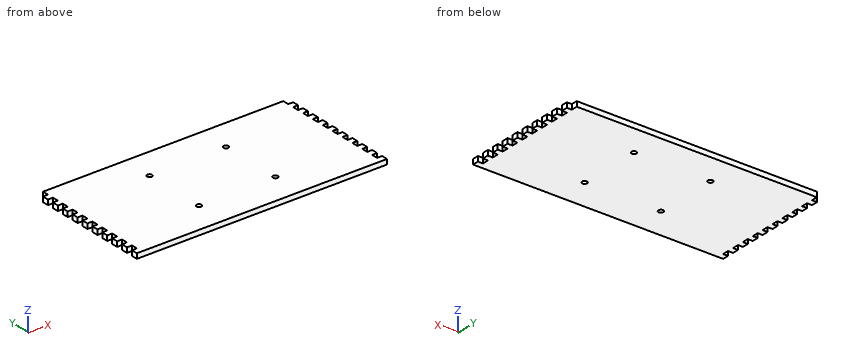
Solid Edge part; units mm, degrees
sketch "Sketch1" plane through (0, 0, 0) normal (0, 0, 1) x (1, 0, 0)
  line L0 (-100, -50) -> (100, -50)
  line L1 (100, -50) -> (100, 50)
  line L2 (100, 50) -> (-100, 50)
  line L3 (-100, 50) -> (-100, -50)
  dimension "D1" = 100
  dimension "D2" = 100
extrude "Protrusion1" add sketch "Sketch1" along normal blind 4
sketch "Sketch2" plane through (14.6999, -33.2226, 4) normal (0, 0, 1) x (1, 0, 0)
  line L0 (-114.6999, 68.2226) -> (-110.6999, 68.2226)
  line L1 (-110.6999, 68.2226) -> (-110.6999, 73.2226)
  line L2 (-110.6999, 73.2226) -> (-114.6999, 73.2226)
  line L3 (-114.6999, 73.2226) -> (-114.6999, 68.2226)
  line L4 (-114.6999, 58.2226) -> (-110.6999, 58.2226)
  line L5 (-110.6999, 58.2226) -> (-110.6999, 63.2226)
  line L6 (-110.6999, 63.2226) -> (-114.6999, 63.2226)
  line L7 (-114.6999, 63.2226) -> (-114.6999, 58.2226)
  line L8 (-114.6999, 48.2226) -> (-110.6999, 48.2226)
  line L9 (-110.6999, 48.2226) -> (-110.6999, 53.2226)
  line L10 (-110.6999, 53.2226) -> (-114.6999, 53.2226)
  line L11 (-114.6999, 53.2226) -> (-114.6999, 48.2226)
  line L12 (-114.6999, 38.2226) -> (-110.6999, 38.2226)
  line L13 (-110.6999, 38.2226) -> (-110.6999, 43.2226)
  line L14 (-110.6999, 43.2226) -> (-114.6999, 43.2226)
  line L15 (-114.6999, 43.2226) -> (-114.6999, 38.2226)
  line L16 (-114.6999, 28.2226) -> (-110.6999, 28.2226)
  line L17 (-110.6999, 28.2226) -> (-110.6999, 33.2226)
  line L18 (-110.6999, 33.2226) -> (-114.6999, 33.2226)
  line L19 (-114.6999, 33.2226) -> (-114.6999, 28.2226)
  line L20 (-114.6999, 18.2226) -> (-110.6999, 18.2226)
  line L21 (-110.6999, 18.2226) -> (-110.6999, 23.2226)
  line L22 (-110.6999, 23.2226) -> (-114.6999, 23.2226)
  line L23 (-114.6999, 23.2226) -> (-114.6999, 18.2226)
  line L24 (-114.6999, 8.2226) -> (-110.6999, 8.2226)
  line L25 (-110.6999, 8.2226) -> (-110.6999, 13.2226)
  line L26 (-110.6999, 13.2226) -> (-114.6999, 13.2226)
  line L27 (-114.6999, 13.2226) -> (-114.6999, 8.2226)
  line L28 (-114.6999, -1.7774) -> (-110.6999, -1.7774)
  line L29 (-110.6999, -1.7774) -> (-110.6999, 3.2226)
  line L30 (-110.6999, 3.2226) -> (-114.6999, 3.2226)
  line L31 (-114.6999, 3.2226) -> (-114.6999, -1.7774)
  line L32 (-114.6999, -11.7774) -> (-110.6999, -11.7774)
  line L33 (-110.6999, -11.7774) -> (-110.6999, -6.7774)
  line L34 (-110.6999, -6.7774) -> (-114.6999, -6.7774)
  line L35 (-114.6999, -6.7774) -> (-114.6999, -11.7774)
  line L36 (-114.6999, 78.2226) -> (-110.6999, 78.2226)
  line L37 (-110.6999, 78.2226) -> (-110.6999, 83.2226)
  line L38 (-110.6999, 83.2226) -> (-114.6999, 83.2226)
  line L39 (-114.6999, 83.2226) -> (-114.6999, 78.2226)
  dimension "D1" = 110.6999
  dimension "D2" = 114.6999
  dimension "D3" = 110.6999
  dimension "D4" = 110.6999
  dimension "D5" = 110.6999
  dimension "D6" = 114.6999
  dimension "D7" = 110.6999
  dimension "D8" = 110.6999
  dimension "D9" = 110.6999
  dimension "D10" = 110.6999
  dimension "D11" = 110.6999
  dimension "D12" = 110.6999
  dimension "D13" = 110.6999
  dimension "D14" = 110.6999
  dimension "D15" = 110.6999
  dimension "D16" = 110.6999
  dimension "D17" = 110.6999
  dimension "D18" = 110.6999
  dimension "D19" = 110.6999
  dimension "D20" = 114.6999
  dimension "D21" = 114.6999
  dimension "D22" = 110.6999
extrude "Cutout1" cut sketch "Sketch2" against normal through all
mirror "Mirror1" about plane through (0, 0, 0) normal (1, 0, 0) of "Cutout1"
hole "Hole_1" at (30.5, 25, 4) direction (0, 0, -1) diameter 4 end through all
hole "Hole1" at (30.5, -25, 4) direction (0, 0, -1) diameter 4 end through all
hole "Hole2" at (-30.5, -25, 4) direction (0, 0, -1) diameter 4 end through all
hole "Hole3" at (-30.5, 25, 4) direction (0, 0, -1) diameter 4 end through all
The model under review builds one solid part; all positions refer to its coordinate system, in mm. Round coordinates to 2 decimals unless told otherwise and drop trailing zeros. Write each loop counter-clockwise with the first axis right and the second up, starting at its lowest first coordinate (ties: lowest second). Pieces come first, ordered by that corner, then holes. Notation, with made-up numbers: M 76,25.25 L 130,25.25 A32 cw 130,61.25 Z; hole C -31,-28 d7. An arc over 180 degrees is marked long. Use CSV: the item, a comma, the result in double quotes. Start each with the question number.
(1) We need section B-B, the plane y = -3. State the section outline as (x, z) points, then the cut area to 3 significant figures.
(2) For line 1 along Y through (x, z) = (30.5, 1.6); line 2 along X through (y, z) = (-25.5, 3.15); line 3 along Y through (x, z) = (29, 1.15), list the stretches that pass through material, from the lowest coordinate up.
(3) We need section C-C, the plane z = 0.6. State how many separate pieces and enclosed holes the cut face has, then the cut area to 3 significant figures.
(4) We need section A-A, the plane x = -30.5. State the section outline as (y, z) points, then the cut area to 3 significant figures.
(5) Clearance check with a flat-ended pin moving along its axis: P1, Ø1.2, axis at y = 18.5, z = 1.5, coming from the +X side. State where the tip first meets the part, or that it passes through.
Findings:
1,outline,"M -96,0 L 96,0 L 96,4 L -96,4 Z"
1,area,"768 mm^2"
2,line 1,"-50 to -27, -23 to 23, 27 to 50"
2,line 2,"-100 to -32.44, -28.56 to 28.56, 32.44 to 100"
2,line 3,"-50 to -26.32, -23.68 to 23.68, 26.32 to 50"
3,separate pieces,"1"
3,enclosed holes,"4"
3,area,"19,500 mm^2"
4,outline,"M -50,0 L -27,0 L -27,4 L -50,4 Z; M -23,0 L 23,0 L 23,4 L -23,4 Z; M 27,0 L 50,0 L 50,4 L 27,4 Z"
4,area,"368 mm^2"
5,P1,"x = 96"
